from build123d import *

# Parameters (mm, degrees)
SKETCH1_W           = 50.8
SKETCH1_H           = 25.4
BOSS_EXTRUDE1_DEPTH = 108.1786
SKETCH2_W           = 44.45
SKETCH2_H           = 19.05
CUT_EXTRUDE1_DEPTH  = 123.181870578
SKETCH3_R           = 12.7
CUT_EXTRUDE2_DEPTH  = 3.175
SKETCH5_R           = 6.35
CUT_EXTRUDE3_DEPTH  = 108.1786


with BuildPart() as part:
    # Sketch1 → Boss-Extrude1 (new body)
    with BuildSketch(Plane.XY):
        with Locations((25.4, -12.7)):
            Rectangle(SKETCH1_W, SKETCH1_H)
    extrude(amount=BOSS_EXTRUDE1_DEPTH)

    # Sketch2 → Cut-Extrude1 (cut, through all)
    with BuildSketch(Plane.XY.offset(108.1786)):
        with Locations((25.4, -12.7)):
            Rectangle(SKETCH2_W, SKETCH2_H)
    extrude(amount=-CUT_EXTRUDE1_DEPTH, mode=Mode.SUBTRACT)

    # Sketch3 → Cut-Extrude2 (cut)
    with BuildSketch(Plane(origin=(0, 0, 0), x_dir=(1, 0, 0), z_dir=(0, 1, 0))):
        with Locations(Location((25.4, -19.2786, 0), (0, 0, 270))):
            Circle(SKETCH3_R)
    extrude(amount=-CUT_EXTRUDE2_DEPTH, mode=Mode.SUBTRACT)

    # Sketch5 → Cut-Extrude3 (cut)
    with BuildSketch(Plane.XZ.offset(25.4)):
        with Locations(Location((25.4, 19.2786, 0), (0, 0, 270))):
            Circle(SKETCH5_R)
    extrude(amount=-CUT_EXTRUDE3_DEPTH, mode=Mode.SUBTRACT)


solid = part.part
Verification items for the finished model (mm, model axes). A direction names the side the tool comes from. Coordinates: 2 decimals unless noted, no trailing zeros. Write each loop counter-clockwise with the first axis right and the second up, starting at its lowest first coordinate (ties: lowest second). Pieces come first, ordered by that corner, then holes. Notation, with made-up numbers: M -21,-25.75 L 37,-25.75 A19 cw 37,-11.75 Z; hole C 54,71 d1. An arc over 180 degrees is marked long. One line per question, with ' | ' between items.
1) Sectioned sample at B-B on y = -11.75. Record the cut outline in (x, z) (3 decimals).
Solutions:
outline: M 0,0 L 3.175,0 L 3.175,108.179 L 0,108.179 Z; M 47.625,0 L 50.8,0 L 50.8,108.179 L 47.625,108.179 Z
2) Material ranges on L1, parallel to X at y = -20.5, z = 60.5 (3 decimals); L2, parallel to Y at x = 10, z = 80.5 (3 decimals); L3, parallel to X at y = -2.5, z = 10, recorded low to high.
Solutions:
L1: 0 to 3.175, 47.625 to 50.8 | L2: -25.4 to -22.225, -3.175 to 0 | L3: 0 to 16.73, 34.07 to 50.8
3) Release check for a two-part mould opening along Y. For faces 4 (the face through (25, -22.225, 55)), 5 (the face through (25, -25.4, 53)), 6 (the face through (25, -2, 108.179)) record: +Y half, -Y half, draft (parallel to the pull), parting line (faces both ways), or undercut.
Solutions:
face 4: undercut | face 5: -Y half | face 6: draft
4) Sectioned sample at A-A on x = 25.4. Record the cut outline in (y, z) (3 decimals).
Solutions:
outline: M -25.4,0 L -22.225,0 L -22.225,12.929 L -25.4,12.929 Z; M -25.4,25.629 L -22.225,25.629 L -22.225,108.179 L -25.4,108.179 Z; M -3.175,0 L 0,0 L 0,6.579 L -3.175,6.579 Z; M -3.175,31.979 L 0,31.979 L 0,108.179 L -3.175,108.179 Z
5) Sectioned sample at D-D on x = 46.5. Record the cut outline in (y, z) (3 decimals), then the cut area to 3 significant figures.
Solutions:
outline: M -25.4,0 L -22.225,0 L -22.225,108.179 L -25.4,108.179 Z; M -3.175,0 L 0,0 L 0,108.179 L -3.175,108.179 Z | area: 687 mm^2
6) Access from +Z, -Z, +X, -X, +Y, -Y to the whole of each face (thin tool, end or side, straight path). Record for faces 1 (the face through (33.983, -1.565, 9.918)), 2 (the face through (3.175, -13, 55)), 3 (the face through (50.8, -13, 53)).
Solutions:
face 1: +Y | face 2: +Z, -Z | face 3: +Z, -Z, +X, +Y, -Y
7) Depth check by flat-ended pin: pin 1 Ø10 at (y, z) = (-21, 58) entering from -X; pin 2 Ø14.5 at (x, z) = (25.4, 19.28) entering from +Y (3 decimals). Enter the tip coordinate at first touch or a pass-through.
Solutions:
pin 1: x = 0 | pin 2: y = -22.225
8) Sectioned sample at C-C on z = 56.5. Record the cut outline in (x, y) (3 decimals).
Solutions:
outline: M 0,-25.4 L 50.8,-25.4 L 50.8,0 L 0,0 Z; hole M 3.175,-22.225 L 47.625,-22.225 L 47.625,-3.175 L 3.175,-3.175 Z
